from build123d import *

# Parameters (mm, degrees)
F0_R     = 50
F1_DEPTH = 140
F2_R     = 50
F2_R_2   = 30
F3_DEPTH = 40
F4_R     = 10
F5_DEPTH = 80


with BuildPart() as f1:
    # F0 (on Front) → F1 (new body)
    with BuildSketch(Plane.XZ):
        Circle(F0_R)
    extrude(amount=F1_DEPTH)

    # F2 (on face) → F3 (join)
    with BuildSketch(Plane.XZ.offset(140)):
        Circle(F2_R)
        Circle(F2_R_2, mode=Mode.SUBTRACT)
    extrude(amount=F3_DEPTH)

    # F4 (on face) → F5 (cut)
    with BuildSketch(Plane.XZ.offset(140)):
        Circle(F4_R)
    extrude(amount=-F5_DEPTH, mode=Mode.SUBTRACT)


solid = f1.part
Work out the finished part from the listing and answer in its coordinate system (mm). A direction names the side the tool comes from. Round coordinates to 2 decimals unless told otherwise and drop trailing zeros. Write each loop counter-clockwise with the first axis right and the second up, starting at its lowest first coordinate (ties: lowest second). Pieces come first, ordered by that corner, then holes.
1) A cutting plane is placed at C-C (z = -15). Give the vertices of the cut face in (x, y).
2) A cutting plane is placed at B-B (z = 17.5). Give the vertices of the cut face in (x, y).
3) Given pin 1 Ø10 at (x, z) = (-4, 2.5) entering from -Y; pin 2 Ø1.5 at (x, z) = (-26, 9.5) entering from -Y; pin 3 Ø12 at (x, y) = (3, -117) entering from -Z, each flat-ended and moving along its own axis, determine where each tip first touches the part or whether it passes through.
4) A tool of negligible diameter and unlimited length cuts with its end or side. For faces 1 (the flat face through (-1, 0, 1)), 2 (the flat face through (13, -140, 0)), from which of +Z, -Z, +X, -X, +Y, -Y can it reach the whole face along a straight path? Write none if from no direction.
5) Straight lines are drawn through the part: line 1 (X direction, y = -123.5, z = 0.5); line 2 (Z direction, x = 0, y = -169). For each, find the intervals that lie inside material, in ascending order.
6) A cutting plane is placed at A-A (x = 0). Give the vertices of the cut face in (y, z), plus the area to 3 significant figures.
7) A cutting plane is placed at D-D (x = 34). Give the vertices of the cut face in (y, z), plus the area to 3 significant figures.
8) The mould has two halves that part along Z. Classify faces 3 (the cylindrical face through (-29.97, -159.72, 1.32)), 4 (the flat face through (0, -60, 0)), 5 (the cylindrical face through (47.69, -88.74, 15.02)), 6 (the flat face through (22, -180, -22)): pulls with the +Z half, pulls with the -Z half, needs draft (parallel to the pull), parting line crosses it, or undercut.
Completed:
1. outline: (-47.7, -180) - (-25.98, -180) - (-25.98, -140) - (25.98, -140) - (25.98, -180) - (47.7, -180) - (47.7, 0) - (-47.7, 0) - close
2. outline: (-46.84, -180) - (-24.37, -180) - (-24.37, -140) - (24.37, -140) - (24.37, -180) - (46.84, -180) - (46.84, 0) - (-46.84, 0) - close
3. pin 1: stops at y = -60
3. pin 2: stops at y = -140
3. pin 3: stops at z = -50
4. face 1: +Z, -Z, +X, -X, +Y
4. face 2: -Y
5. line 1: x = -50 to -9.99, 9.99 to 50
5. line 2: z = -50 to -30, 30 to 50
6. outline: (-180, -50) - (0, -50) - (0, 50) - (-180, 50) - (-180, 30) - (-140, 30) - (-140, 10) - (-60, 10) - (-60, -10) - (-140, -10) - (-140, -30) - (-180, -30) - close
6. area: 14,000 mm2
7. outline: (-180, -36.66) - (0, -36.66) - (0, 36.66) - (-180, 36.66) - close
7. area: 13,200 mm2
8. face 3: undercut
8. face 4: undercut
8. face 5: parting line crosses it
8. face 6: needs draft
